from build123d import *

# Parameters (mm, degrees)
DODANIE_WYCI_GNI_CIE1_DEPTH      = 1
DODANIE_WYCI_GNI_CIE1_DEPTH_BACK = 9.9


with BuildPart() as part:
    # Szkic1 → Dodanie-wyciągnięcie1 (new body, two sides)
    with BuildSketch(Plane.XY) as dodanie_wyci_gni_cie1_sk:
        with BuildLine():
            Line((-250, -49), (0, -49))
            ThreePointArc((0, -49), (49, 0), (0, 49))
            Line((0, 49), (-250, 49))
            ThreePointArc((-250, 49), (-299, 0), (-250, -49))
        make_face()
        with BuildLine():
            ThreePointArc((0, 40.63), (40.63, 0), (0, -40.63))
            Line((0, -40.63), (-0.2047739, -40.62948397))
            Line((-0.2047739, -40.62948397), (-242.972914826, -40.017708255))
            ThreePointArc((-242.972914826, -40.017708255), (-290.476637622, -3.526855087), (-250, 40.63))
            Line((-250, 40.63), (0, 40.63))
        make_face(mode=Mode.SUBTRACT)
    extrude(amount=DODANIE_WYCI_GNI_CIE1_DEPTH)
    extrude(dodanie_wyci_gni_cie1_sk.sketch, amount=-DODANIE_WYCI_GNI_CIE1_DEPTH_BACK)


solid = part.part
Check sheet for the modelled part. Datum: model origin and axes. Units: mm. A direction names the side the tool comes from. Round coordinates to 2 decimals unless told otherwise and drop trailing zeros. Write each loop counter-clockwise with the first axis right and the second up, starting at its lowest first coordinate (ties: lowest second). Pieces come first, ordered by that corner, then holes. Notation, with made-up numbers: (13, 48.5) - (69, 48.5) arc R34 cw to (69, 80.5) - close; hole circle Ø7 at (61, 6). An arc over 180 degrees is marked (long way). Return JSON: item names as keys, results as strings.
Q1. Scan lines: L1, parallel to X at y = 0, z = -2.75; L2, parallel to Y at x = -250, z = -6.5; L3, parallel to X at y = 21.5, z = -6. Record each from-to range of solid material in increasing order. Write a range as from..to.
Returned:
{"L1": "x = -299..-290.63, 40.63..49", "L2": "y = -49..-40.63, 40.63..49", "L3": "x = -294.03..-284.48, 34.48..44.03"}
Q2. Depth check by flat-ended pin: P1, Ø5, axis at y = -24.5, z = -1, coming from the +X side; P2, Ø2, axis at y = -23.5, z = -5.5, coming from the +X side. Enter the tip coordinate at first touch or a pass-through.
Returned:
{"P1": "stops at x = 43.78", "P2": "stops at x = 43.53"}
Q3. Cross-section at C-C (x = -231). Record the boundary of the cut face in (y, z).
Returned:
{"outline": "(-49, -9.9) - (-40.05, -9.9) - (-40.05, 1) - (-49, 1) - close; (40.63, -9.9) - (49, -9.9) - (49, 1) - (40.63, 1) - close"}
Q4. Draft check along Y on faces 1 (the flat face through (-127, -49, -4)), 2 (the flat face through (-127, 40.63, -4)), 3 (the flat face through (-126, -43, -9.9)), 4 (the cylindrical face through (48.99, -1.08, -4.37)). Enter one of: released by +Y, released by -Y, zero draft, split by the parting line, or undercut.
Returned:
{"face 1": "released by -Y", "face 2": "undercut", "face 3": "zero draft", "face 4": "split by the parting line"}
Q5. Cross-section at A-A (y = 0). Record the boundary of the cut face in (x, z), then the cut area to 3 significant figures.
Returned:
{"outline": "(-299, -9.9) - (-290.63, -9.9) - (-290.63, 1) - (-299, 1) - close; (40.63, -9.9) - (49, -9.9) - (49, 1) - (40.63, 1) - close", "area": "182 mm²"}
Q6. Access from +Z, -Z, +X, -X, +Y, -Y to the whole of each face (thin tool, end or side, straight path). Record for faces 5 (the cylindrical face through (-298.99, 1.08, -4.37)), 6 (the cylindrical face through (40.62, 0.89, -4.37)).
Returned:
{"face 5": "+Z, -Z, -X", "face 6": "+Z, -Z"}
Q7. Cross-section at B-B (z = -6.25). Record the boundary of the cut face in (x, y), then the cut area to 3 significant figures.
Returned:
{"outline": "(-250, -49) - (0, -49) arc R49 ccw to (0, 49) - (-250, 49) arc R49 ccw to start; hole (-250, 40.63) arc R40.63 ccw (long way) to (-242.97, -40.02) - (0, -40.63) arc R40.63 ccw to (0, 40.63) - close", "area": "6,620 mm²"}
